Source: three-view drawing plus pictorial views. Frame: mm from the lowest corner of the part. A direction names the side the tool comes from. Give positions to 0.01 mm unless a question says otherwise; leave off trailing zeros. Loops run counter-clockwise (first coordinate to the right, second up) from the corner with the lowest first, then second, coordinate; pieces in that order, holes last.
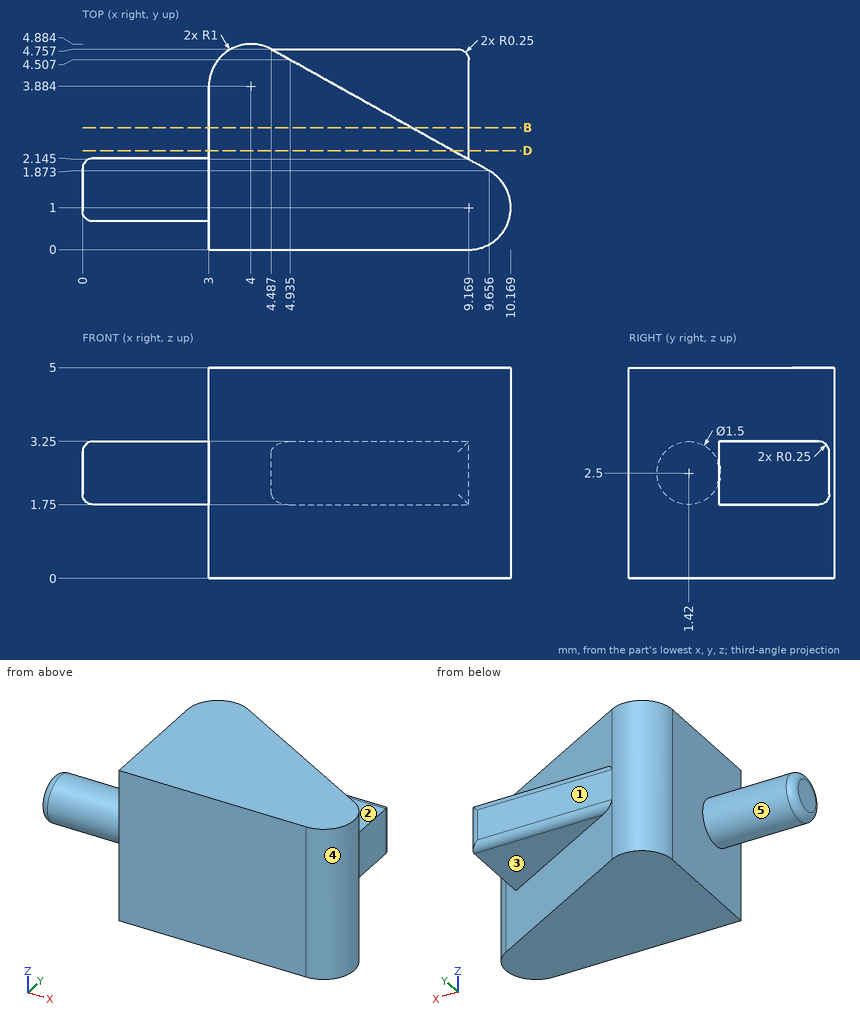
1) Cut plane D-D (y = 2.35). Return loops of the section in (x, z).
Checks:
outline: (3, 0) - (8.8, 0) - (8.8, 1.75) - (9.17, 1.75) - (9.17, 3.25) - (8.8, 3.25) - (8.8, 5) - (3, 5) - close
2) Ray query, probe 1 along Z at (x, y) = (6.75, 3.6); probe 2 along Y at (x, z) = (4.5, 2.25); probe 3 along X at (y, z) = (4.1, 3.1). Return the intervals inside material, ascending.
Checks:
probe 1: z = 1.75 to 3.25
probe 2: y = 0 to 4.76
probe 3: x = 3.02 to 9.17
3) Reachability of the marked faces 1, 2, 3, 4 and 5 from +Z, -Z, +X, -X, +Y, -Y: full face, straight path, thin tool, end or side. Return the list, or none.
Checks:
face 1: +Z, -Z, +X, +Y
face 2: +Z, +X, +Y
face 3: -Z, +X, +Y
face 4: +Z, -Z, +X
face 5: -X
4) Cut plane B-B (y = 2.9). Return loops of the section in (x, z).
Checks:
outline: (3, 0) - (7.82, 0) - (7.82, 1.75) - (9.17, 1.75) - (9.17, 3.25) - (7.82, 3.25) - (7.82, 5) - (3, 5) - close
5) Contact query for flat-ended pins moving along their axis: P1, Ø1.9, axis at y = 1.5, z = 3.5, coming from the -X side; P2, Ø1.6, axis at y = 3, z = 3, coming from the +X side. Output: stop coordinate, or through.
Checks:
P1: stops at x = 0
P2: stops at x = 9.17
